Print and shaded views of the part. All mm, measured from the part's lowest x, y and z. Round coordinates to 2 decimals unless told otherwise and drop trailing zeros. Order: outer loops, then holes, each group sorted by start corner. A loop starts at its lowest first (then second) coordinate and runs counter-clockwise, first axis right, second up. Notation, with made-up numbers: (52.5, 77.25) -> (101.5, 77.25) arc R35 cw to (101.5, 113.25) -> close; hole circle Ø10 at (38, -37.75). An arc over 180 degrees is marked (long way). Answer as CSV lines item,"result".
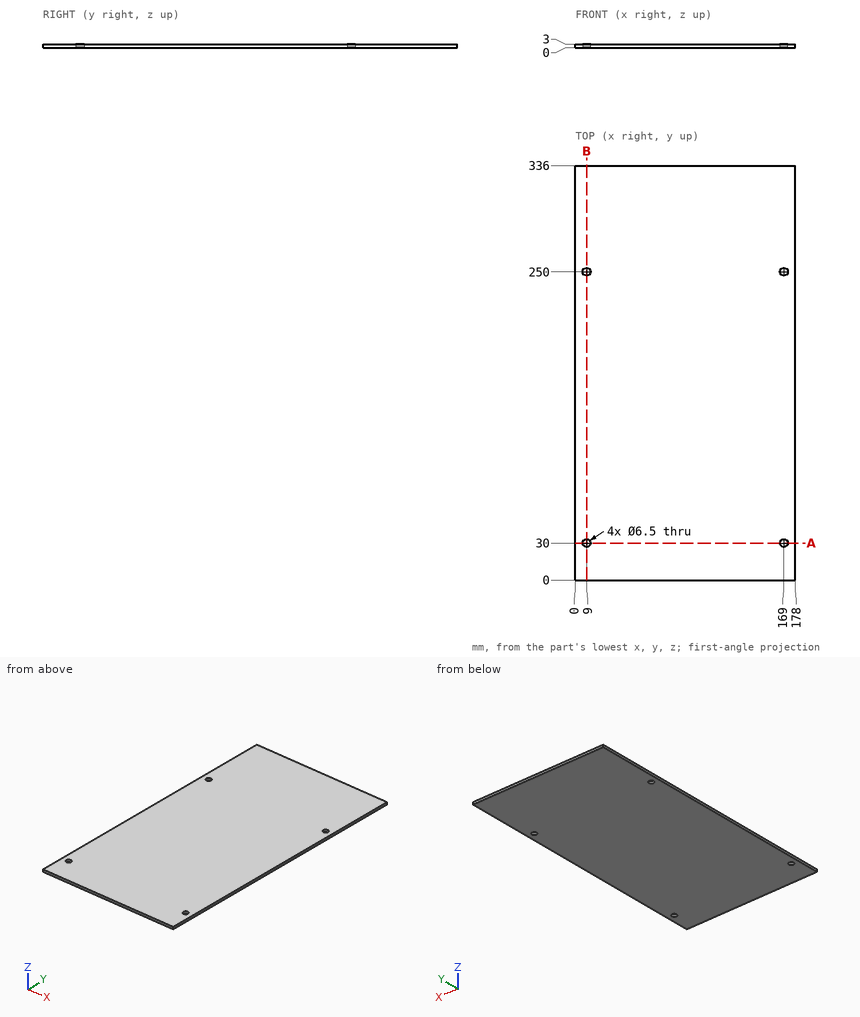
Q1. Wall check: L1, parallel to X at y = 250, z = 0.8; L2, parallel to Y at x = 9, z = 1.2; L3, parallel to X at y = 253, z = 1.55. Give the ranges that are in metal, low to high. Write a range as [from, to].
Checks:
L1,"[0, 5.75], [12.25, 165.75], [172.25, 178]"
L2,"[0, 26.75], [33.25, 246.75], [253.25, 336]"
L3,"[0, 7.75], [10.25, 167.75], [170.25, 178]"
Q2. Saw through at B-B (x = 9). Write the cut outline in (y, z).
Checks:
outline,"(0, 0) -> (26.75, 0) -> (26.75, 3) -> (0, 3) -> close; (33.25, 0) -> (246.75, 0) -> (246.75, 3) -> (33.25, 3) -> close; (253.25, 0) -> (336, 0) -> (336, 3) -> (253.25, 3) -> close"
Q3. Saw through at A-A (y = 30). Write the cut outline in (x, z), plus the area to 3 significant figures.
Checks:
outline,"(0, 0) -> (5.75, 0) -> (5.75, 3) -> (0, 3) -> close; (12.25, 0) -> (165.75, 0) -> (165.75, 3) -> (12.25, 3) -> close; (172.25, 0) -> (178, 0) -> (178, 3) -> (172.25, 3) -> close"
area,"495 mm²"
